Could you check a few things on this model? Use its own coordinates, in mm. A direction names the side the tool comes from. Give positions to 0.01 mm unless a question says otherwise; leave off trailing zeros. Loops run counter-clockwise (first coordinate to the right, second up) from the corner with the lowest first, then second, coordinate; pieces in that order, holes last. Notation, with made-up numbers: (-20, -4.75) - (2, -4.75) arc R18 ccw to (2, 5.25) - close; hole circle Ø2 at (63, -6). An arc over 180 degrees is marked (long way). Use CSV: the item, a comma, the result in double quotes.
Autodesk Inventor part; units mm, degrees
ref_plane "YZ Plane" through (0, 0, 0) normal (1, 0, 0) x (0, 1, 0)
ref_plane "XZ Plane" through (0, 0, 0) normal (0, 1, 0) x (-1, 0, 0)
ref_plane "XY Plane" through (0, 0, 0) normal (0, 0, 1) x (1, 0, 0)
sketch "Sketch1" plane through (0, 0, 0) normal (0, 0, 1) x (1, 0, 0)
  line L0 (0, 0) -> (76.2, 0)
  line L1 (76.2, 0) -> (76.2, 50.8)
  line L2 (76.2, 50.8) -> (0, 50.8)
  line L3 (0, 50.8) -> (0, 0)
  dimension "d0" = 76.2
  dimension "d1" = 50.8
extrude "Extrusion1" add sketch "Sketch1" along normal blind 1219.2
shell "Shell1" thickness 3.175 removed faces 2 at (50.8, 16.9333, 0) at (50.8, 16.9333, 1219.2)
fillet "Fillet1" radius 3.175 8 edges at (0, 50.8, 609.6) (3.175, 3.175, 609.6) (73.025, 3.175, 609.6) (3.175, 47.625, 609.6) (73.025, 47.625, 609.6) (76.2, 50.8, 609.6) (0, 0, 609.6) (76.2, 0, 609.6)
properties part number "2x3_Tube"
1) Which directions (+Z, -Z, +X, -X, +Y, -Y) give clear straight access to the entire face, cutting with the end or side of a thin tool? Please do faces 1 (the flat face through (3.175, 26, 601)), 2 (the flat face through (35, 3, 1219.2)).
Answer below:
face 1,"+Z, -Z"
face 2,"+Z, +X, -X, +Y, -Y"
2) Suppose I cut it at A-A (y = 29). Please give me the cut outline in (x, z) (3 decimals), plus the area to 3 significant figures.
Answer below:
outline,"(0, 0) - (3.175, 0) - (3.175, 1219.2) - (0, 1219.2) - close; (73.025, 0) - (76.2, 0) - (76.2, 1219.2) - (73.025, 1219.2) - close"
area,"7,740 mm2"
3) I need wall thicknesses on line 1 along X through (y, z) = (28.5, 449.5) (3 decimals); line 2 along Y through (x, z) = (59, 487) (3 decimals); line 3 along X through (y, z) = (47, 885). Which ranges of each line are inside material? Lowest first, please.
Answer below:
line 1,"x = 0 to 3.175, 73.025 to 76.2"
line 2,"y = 0 to 3.175, 47.625 to 50.8"
line 3,"x = 0 to 4.46, 71.74 to 76.2"
4) Suppose I cut it at C-C (x = 29.5). Please give me the cut outline in (y, z) (3 decimals), plus the area to 3 significant figures.
Answer below:
outline,"(0, 0) - (3.175, 0) - (3.175, 1219.2) - (0, 1219.2) - close; (47.625, 0) - (50.8, 0) - (50.8, 1219.2) - (47.625, 1219.2) - close"
area,"7,740 mm2"
5) Suppose I cut it at B-B (z = 477.5). Please give me the cut outline in (x, y) (3 decimals).
Answer below:
outline,"(0, 3.175) arc R3.175 ccw to (3.175, 0) - (73.025, 0) arc R3.175 ccw to (76.2, 3.175) - (76.2, 47.625) arc R3.175 ccw to (73.025, 50.8) - (3.175, 50.8) arc R3.175 ccw to (0, 47.625) - close; hole (3.175, 6.35) arc R3.175 ccw to (6.35, 3.175) - (69.85, 3.175) arc R3.175 ccw to (73.025, 6.35) - (73.025, 44.45) arc R3.175 ccw to (69.85, 47.625) - (6.35, 47.625) arc R3.175 ccw to (3.175, 44.45) - close"
6) We'd pull the mould along X, two halves only. Please class faces 3 (the flat face through (39, 47.625, 601)), 4 (the flat face through (35, 3, 0)), 5 (the flat face through (0, 26, 601)): +X half, -X half, draft (parallel to the pull), parting line (faces both ways), or undercut.
Answer below:
face 3,"undercut"
face 4,"draft"
face 5,"-X half"
